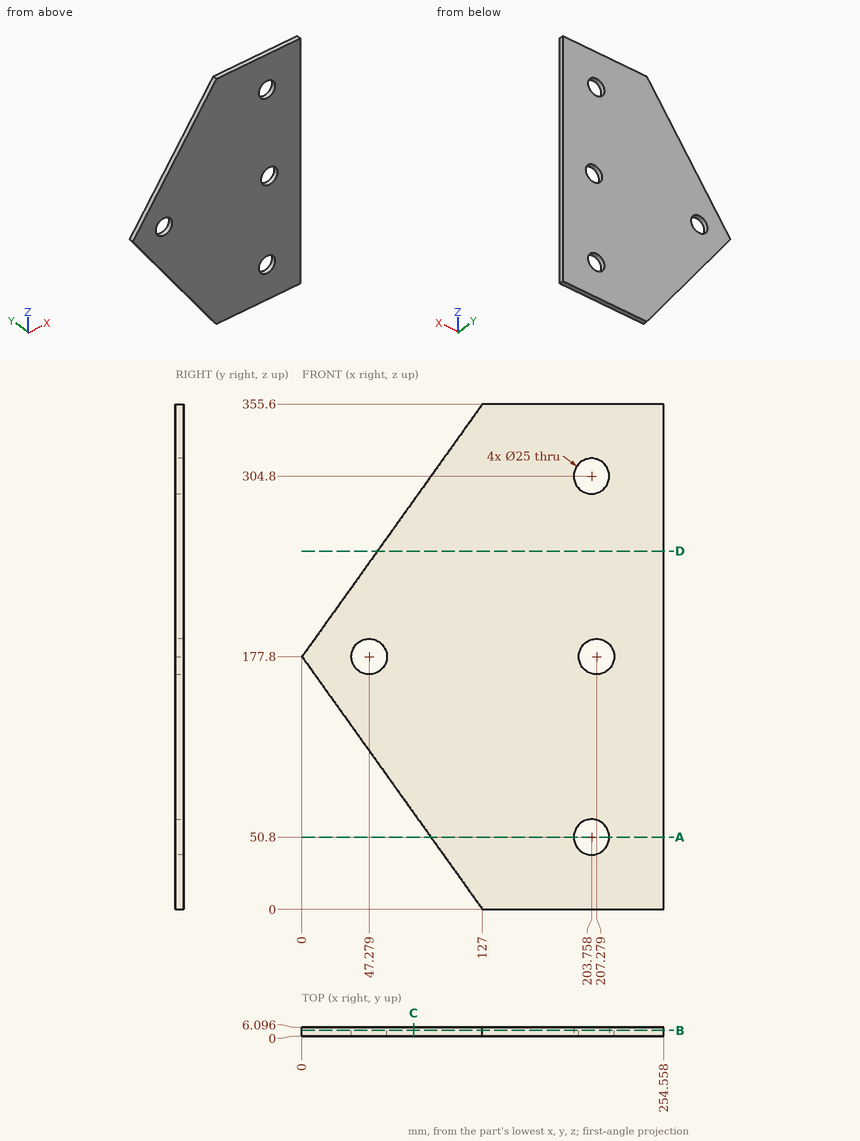
Geometry check sheet. Reference: drawing and pictorial views, mm from the part's lowest x, y, z. Give positions to 0.01 mm unless a question says otherwise; leave off trailing zeros. Loops run counter-clockwise (first coordinate to the right, second up) from the corner with the lowest first, then second, coordinate; pieces in that order, holes last. Notation, with made-up numbers: M 23.25,53.5 L 52.25,53.5 A12 cw 52.25,63.5 Z; hole C -5.75,56.5 d10. An arc over 180 degrees is marked long. Use a Markdown table: item, result. Add a question column.
Q1. Go/stop test with flat-tipped pins: pin 1 (1 mm diameter, centred on y = 3, z = 318.5, fed in from -X); pin 2 (1 mm diameter, centred on x = 72, y = 3, fed in from -Z); pin 3 (22.5 mm diameter, centred on x = 203.76, z = 304.8, fed in from +Y); pin 4 (3 mm diameter, centred on x = 66.5, y = 0.5, fed in from +Z). Record where each tip stops, or that it passes through.
Q2. Scan lines: line 1 along X through (y, z) = (4, 177.8); line 2 along X through (y, z) = (2.25, 304.8) (1 decimal); line 3 along Z through (x, y) = (40, 5.5) (1 decimal). Record each from-to range of solid material in increasing order. Write a range as [from, to].
Q3. Sectioned sample at A-A, the plane z = 50.8. Record the cut outline in (x, y) (1 decimal).
Q4. Sectioned sample at D-D, the plane z = 252. Record the cut outline in (x, y), then the cut area to 3 significant figures.
Q5. Sectioned sample at B-B, the plane y = 4. Record the cut outline in (x, z).
Q6. Sectioned sample at C-C, the plane x = 78.5. Record the cut outline in (y, z).
Verdict:
| question | item | result |
|---|---|---|
| 1 | pin 1 | x = 100.14 |
| 1 | pin 2 | z = 76.3 |
| 1 | pin 3 | through |
| 1 | pin 4 | z = 273 |
| 2 | line 1 | [0, 34.78], [59.78, 194.78], [219.78, 254.56] |
| 2 | line 2 | [90.7, 191.3], [216.3, 254.6] |
| 2 | line 3 | [121.8, 167.6], [188, 233.8] |
| 3 | outline | M 90.7,0 L 191.3,0 L 191.3,6.1 L 90.7,6.1 Z; M 216.3,0 L 254.6,0 L 254.6,6.1 L 216.3,6.1 Z |
| 4 | outline | M 53,0 L 254.56,0 L 254.56,6.1 L 53,6.1 Z |
| 4 | area | 1,230 mm^2 |
| 5 | outline | M 0,177.8 L 127,0 L 254.56,0 L 254.56,355.6 L 127,355.6 Z; hole C 47.28,177.8 d25; hole C 203.76,50.8 d25; hole C 203.76,304.8 d25; hole C 207.28,177.8 d25 |
| 6 | outline | M 0,67.9 L 6.1,67.9 L 6.1,287.7 L 0,287.7 Z |
